Source: three-view drawing plus pictorial views. Frame: mm from the lowest corner of the part. Give positions to 0.01 mm unless a question says otherwise; leave off trailing zeros. Order: outer loops, then holes, each group sorted by start corner. A loop starts at its lowest first (then second) coordinate and runs counter-clockwise, first axis right, second up. Notation, with made-up numbers: (48, 60.5) - (102, 60.5) arc R11 cw to (102, 76.5) - close; hole circle Ø9 at (79.25, 25). An arc over 180 degrees is marked (long way). Use one line per item in the form item = value.
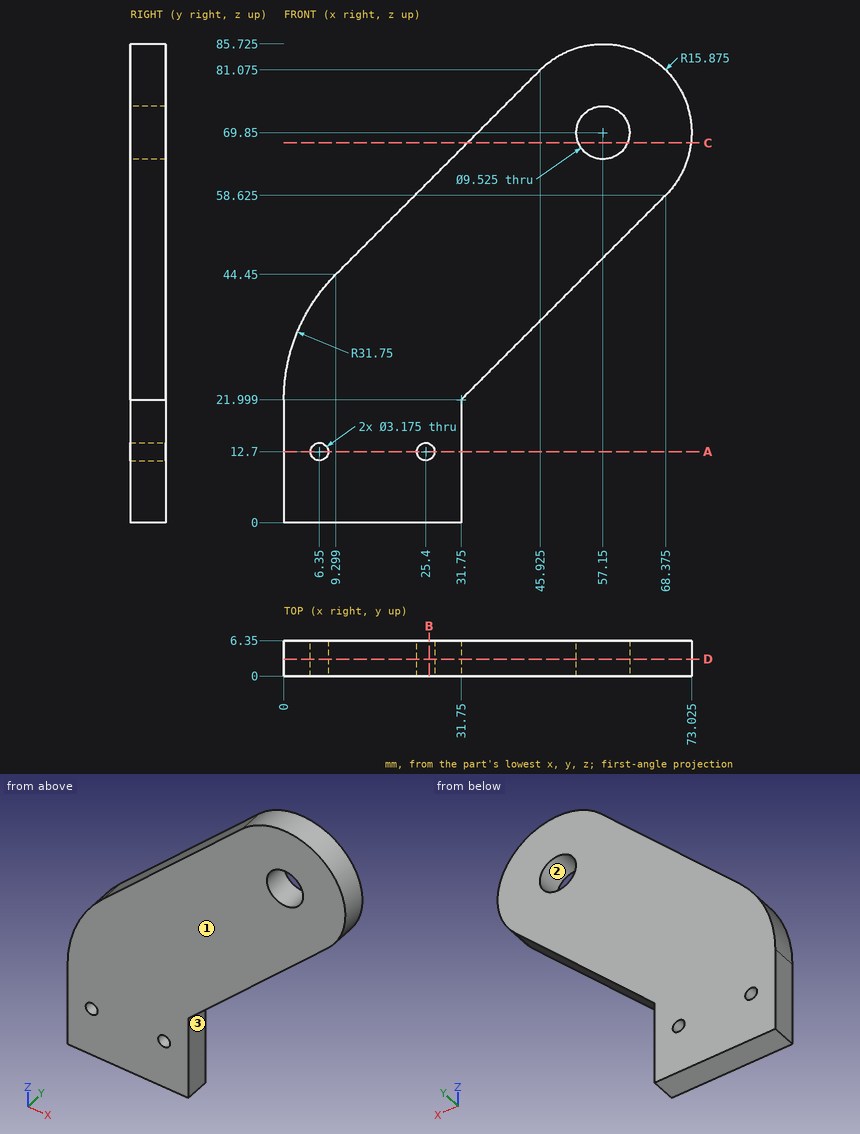
(1) Pull-direction query (X, two-part tool) for the marked faces 1, 2 and 3; classes: released by +X, released by -X, zero draft, split by the parting line, or undercut.
Computed values:
face_1 = zero draft
face_2 = undercut
face_3 = released by +X
(2) Cut plane B-B on x = 26. Output: boundary loops of the cut face in (y, z), plus the area to 3 significant figures.
Computed values:
outline = (0, 0) - (6.35, 0) - (6.35, 11.23) - (0, 11.23) - close; (0, 14.17) - (6.35, 14.17) - (6.35, 61.15) - (0, 61.15) - close
area = 370 mm²
(3) Contact query for flat-ended pins moving along their axis: pin 1 Ø1.9 at (y, z) = (3, 13) entering from +X; pin 2 Ø1.5 at (y, z) = (4.5, 39) entering from -X (1 decimal). Output: stop coordinate, or through.
Computed values:
pin_1 = 31.75
pin_2 = 4.5
(4) Cut plane A-A on z = 12.7. Output: boundary loops of the cut face in (x, y).
Computed values:
outline = (0, 0) - (4.76, 0) - (4.76, 6.35) - (0, 6.35) - close; (7.94, 0) - (23.81, 0) - (23.81, 6.35) - (7.94, 6.35) - close; (26.99, 0) - (31.75, 0) - (31.75, 6.35) - (26.99, 6.35) - close
(5) Ray query, line 1 along X through (y, z) = (3, 12.7); line 2 along X through (y, z) = (4.5, 6); line 3 along Z through (x, y) = (57.15, 1.75) (1 decimal). Return the intervals inside material, ascending.
Computed values:
line_1 = 0 to 4.76, 7.94 to 23.81, 26.99 to 31.75
line_2 = 0 to 31.75
line_3 = 47.4 to 65.1, 74.6 to 85.7
(6) Cut plane C-C on z = 68. Output: boundary loops of the cut face in (x, y), plus the area to 3 significant figures.
Computed values:
outline = (32.85, 0) - (52.76, 0) - (52.76, 6.35) - (32.85, 6.35) - close; (61.54, 0) - (72.92, 0) - (72.92, 6.35) - (61.54, 6.35) - close
area = 199 mm²
(7) Cut plane D-D on y = 3. Give the number of separate pieces and of enclosed holes in the cut face, plus the area to 3 significant figures.
Computed values:
separate_pieces = 1
enclosed_holes = 3
area = 3,050 mm²
